Input: part model. Units: mm. Frame: model coordinates. A direction names the side the tool comes from. Coordinates: 2 decimals unless noted, no trailing zeros. Loops run counter-clockwise (first coordinate to the right, second up) from the corner with the lowest first, then second, coordinate; pieces in that order, holes last. Notation, with made-up numbers: M 34.5,72.5 L 48.5,72.5 A18 cw 48.5,103.5 Z; hole C 80.25,-16 d5. An arc over 180 degrees is marked long. Use a Markdown table: item, result. Add a question column.
1. Draft query along X for faces 1 (the flat face through (0.2, 0.5, -0.6)), 2 (the cylindrical face through (0, 5, 1)), 3 (the flat face through (1, 1.6, 1)). Return one class per face: +X half, -X half, draft (parallel to the pull), parting line (faces both ways), or undercut.
2. Section C-C on y = 2. Output: boundary loops of the cut face in (x, z), then the cut area to 3 significant figures.
3. Section A-A on z = 0. Output: boundary loops of the cut face in (x, y).
4. Pin query (flat end, axial travel): pin 1 (1.5 mm diameter, centred on y = 4, z = -0.5, fed in from -X); pin 2 (0.9 mm diameter, centred on y = 0.5, z = -0.5, fed in from +X); pin 3 (2 mm diameter, centred on y = 6.5, z = 1.5, fed in from -X). Return the tip coordinate at first contact, or that it passes through.
5. Section D-D on x = -1.1. Output: boundary loops of the cut face in (y, z).
6. Line query: L1, parallel to X at y = 7, z = -0.05; L2, parallel to Y at x = 0.15, z = 0.05; L3, parallel to X at y = 0.5, z = 0.7. Output: solid intervals per line, ascending. Write a range as [from, to].
7. Section B-B on x = 0. Output: boundary loops of the cut face in (y, z).
8. Set-up query: faces 4 (the cylindrical face through (1.908, 1.184, -0.601)), 5 (the flat face through (0.2, 0.5, 0.6)). Return all of +Z, -Z, +X, -X, +Y, -Y with unobstructed straight access to the full face (end or side cutting, diameter ignored); none if empty.
```python
from build123d import *

# Parameters (mm, degrees)
SKETCH_1_R          = 2
EXTRUDE_1_DEPTH     = 1.6
SKETCH_2_R          = 1
EXTRUDE_2_DEPTH     = 6
CUT_EXTRUDE_1_DEPTH = 6


with BuildPart() as part:
    # 草图1 → 凸台-拉伸1 (new body)
    with BuildSketch(Plane(origin=(0, 0, 0), x_dir=(1, 0, 0), z_dir=(0, 1, 0))):
        Circle(SKETCH_1_R)
    extrude(amount=EXTRUDE_1_DEPTH)

    # 草图2 → 凸台-拉伸2 (add)
    with BuildSketch(Plane(origin=(0, 1.6, 0), x_dir=(1, 0, 0), z_dir=(0, 1, 0))):
        Circle(SKETCH_2_R)
    extrude(amount=EXTRUDE_2_DEPTH)

    # 草图3 one side → 切除-旋转3 (revolve, cut)
    with BuildSketch(Plane(origin=(0, 0, 0), x_dir=(0, 0, -1), z_dir=(1, 0, 0))):
        with BuildLine():
            ThreePointArc((2, 0.779106216), (1.073196918, 0.201653394), (0, 0))
            Line((0, 0), (0, -0.936416285))
            Line((0, -0.936416285), (3.543500435, -0.936416285))
            Line((3.543500435, -0.936416285), (2, 0.779106216))
        make_face()
    revolve(axis=Axis((0, 1.035939113, 0), (0, -1, 0)), mode=Mode.SUBTRACT)

    # 草图4 → 切除-拉伸1 (cut)
    with BuildSketch(Plane(origin=(0, -5, 0), x_dir=(1, 0, 0), z_dir=(0, 1, 0))):
        Polygon((-1, -0.2), (-0.2, -0.2), (-0.2, -1), (0.2, -1), (0.2, -0.2), (1, -0.2), (1, 0.2), (0.2, 0.2), (0.2, 1), (-0.2, 1), (-0.2, 0.2), (-1, 0.2), align=None)
    extrude(amount=CUT_EXTRUDE_1_DEPTH, mode=Mode.SUBTRACT)


solid = part.part
```
Answers below:
| question | item | result |
|---|---|---|
| 1 | face 1 | undercut |
| 1 | face 2 | parting line |
| 1 | face 3 | draft |
| 2 | outline | C 0,0 d2 |
| 2 | area | 3.14 mm² |
| 3 | outline | M -2,0.78 A2.96 ccw -1,0.17 L -1,1 L 1,1 L 1,0.17 A2.96 ccw 2,0.78 L 2,1.6 L 1,1.6 L 1,7.6 L -1,7.6 L -1,1.6 L -2,1.6 Z |
| 4 | pin 1 | stops at x = -1 |
| 4 | pin 2 | stops at x = 1.99 |
| 4 | pin 3 | stops at x = -0.87 |
| 5 | outline | M 0.78,-1.67 L 1.6,-1.67 L 1.6,1.67 L 0.78,1.67 A2.74 ccw Z |
| 6 | L1 | x = [-1, 1] |
| 6 | L2 | y = [1, 7.6] |
| 6 | L3 | x = [-1.49, -0.2], [0.2, 1.49] |
| 7 | outline | M 0.17,-1 A2.96 ccw 0.78,-2 L 1.6,-2 L 1.6,-1 L 7.6,-1 L 7.6,1 L 1.6,1 L 1.6,2 L 0.78,2 A2.96 ccw 0.17,1 L 1,1 L 1,-1 Z |
| 8 | face 4 | +Y, -Y |
| 8 | face 5 | -Y |
